```python
from build123d import *

# Parameters (mm, degrees)
CROQUIS1_W              = 125
CROQUIS1_H              = 70
SALIENTE_EXTRUIR1_DEPTH = 3
CROQUIS2_W              = 10
CROQUIS2_H              = 2
CORTAR_EXTRUIR1_DEPTH   = 10
CROQUIS3_W              = 31
CROQUIS3_H              = 2
CORTAR_EXTRUIR2_DEPTH   = 10
CROQUIS4_W              = 11
CROQUIS4_H              = 10
CORTAR_EXTRUIR3_DEPTH   = 10


with BuildPart() as part:
    # Croquis1 → Saliente-Extruir1 (new body)
    with BuildSketch(Plane(origin=(0, 0, 0), x_dir=(1, 0, 0), z_dir=(0, 1, 0))):
        Rectangle(CROQUIS1_W, CROQUIS1_H)
    extrude(amount=SALIENTE_EXTRUIR1_DEPTH)

    # Croquis2 → Cortar-Extruir1 (cut)
    with BuildSketch(Plane(origin=(0, 3, 0), x_dir=(1, 0, 0), z_dir=(0, 1, 0))):
        with Locations((-56, 29.2)):
            Rectangle(CROQUIS2_W, CROQUIS2_H)
        with Locations((56, 29.2)):
            Rectangle(CROQUIS2_W, CROQUIS2_H)
    extrude(amount=-CORTAR_EXTRUIR1_DEPTH, mode=Mode.SUBTRACT)

    # Croquis3 → Cortar-Extruir2 (cut)
    with BuildSketch(Plane(origin=(0, 3, 0), x_dir=(1, 0, 0), z_dir=(0, 1, 0))):
        with Locations((0, -30.5)):
            Rectangle(CROQUIS3_W, CROQUIS3_H)
    extrude(amount=-CORTAR_EXTRUIR2_DEPTH, mode=Mode.SUBTRACT)

    # Croquis4 → Cortar-Extruir3 (cut)
    with BuildSketch(Plane(origin=(0, 3, 0), x_dir=(1, 0, 0), z_dir=(0, 1, 0))):
        with Locations((-27, -8)):
            Rectangle(CROQUIS4_W, CROQUIS4_H)
        with Locations((27, -8)):
            Rectangle(CROQUIS4_W, CROQUIS4_H)
    extrude(amount=-CORTAR_EXTRUIR3_DEPTH, mode=Mode.SUBTRACT)


solid = part.part
```
The listing builds one solid part. Answer for the finished solid, in the listing's coordinates (mm). A direction names the side the tool comes from. Give positions to 0.01 mm unless a question says otherwise; leave off trailing zeros. Order: outer loops, then holes, each group sorted by start corner. A loop starts at its lowest first (then second) coordinate and runs counter-clockwise, first axis right, second up. Notation, with made-up numbers: (15, 89.25) -> (32, 89.25) arc R15 ccw to (32, 101.25) -> close; hole circle Ø10 at (21.5, 11.5). An arc over 180 degrees is marked (long way). Answer as a JSON object with one key per item and string values. Group by question number.
Item 1: The part is cut by section A-A on x = 8.5. Write down the section's boundary in (y, z), and give its area (3 significant figures).
Item 2: Determine the mould class of faces 3 (the flat face through (-62.5, 1, 0)), 4 (the flat face through (-1, 3, 0)), 5 (the flat face through (-32.5, 2, 8)) for opening direction X: pulls with the +X half, pulls with the -X half, needs draft (parallel to the pull), parting line crosses it, or undercut.
Item 3: The part is cut by section B-B on z = 9. Write down the section's boundary in (x, y), and give its area (3 significant figures).
Item 4: A tool of negligible diameter and unlimited length cuts with its end or side. For faces 1 (the flat face through (56, 2, -30.2)), 2 (the flat face through (-1, 1, -35)), from which of +Z, -Z, +X, -X, +Y, -Y can it reach the whole face along a straight path? Write none if from no direction.
Item 5: Consider L1, parallel to X at y = 0.6, z = 5; L2, parallel to Z at x = -30, y = 1.15; L3, parallel to Z at x = 8.5, y = 1.55. Determine where each line is inside the solid, lowest interval first. Write a range as from..to.
Item 6: The part is cut by section C-C on y = 0.9. Write down the section's boundary in (x, z).
Result set:
{
 "1": {"outline": "(0, -35) -> (3, -35) -> (3, 29.5) -> (0, 29.5) -> close; (0, 31.5) -> (3, 31.5) -> (3, 35) -> (0, 35) -> close", "area": "204 mm²"},
 "2": {"face 3": "pulls with the -X half", "face 4": "needs draft", "face 5": "undercut"},
 "3": {"outline": "(-62.5, 0) -> (-32.5, 0) -> (-32.5, 3) -> (-62.5, 3) -> close; (-21.5, 0) -> (21.5, 0) -> (21.5, 3) -> (-21.5, 3) -> close; (32.5, 0) -> (62.5, 0) -> (62.5, 3) -> (32.5, 3) -> close", "area": "309 mm²"},
 "4": {"face 1": "+Y, -Y", "face 2": "-Z, +X, -X, +Y, -Y"},
 "5": {"L1": "-62.5..-32.5, -21.5..21.5, 32.5..62.5", "L2": "-35..3, 13..35", "L3": "-35..29.5, 31.5..35"},
 "6": {"outline": "(-62.5, -35) -> (62.5, -35) -> (62.5, 35) -> (-62.5, 35) -> close; hole (-61, -30.2) -> (-51, -30.2) -> (-51, -28.2) -> (-61, -28.2) -> close; hole (-32.5, 3) -> (-21.5, 3) -> (-21.5, 13) -> (-32.5, 13) -> close; hole (-15.5, 29.5) -> (15.5, 29.5) -> (15.5, 31.5) -> (-15.5, 31.5) -> close; hole (21.5, 3) -> (32.5, 3) -> (32.5, 13) -> (21.5, 13) -> close; hole (51, -30.2) -> (61, -30.2) -> (61, -28.2) -> (51, -28.2) -> close"}
}
